Input: part model. Units: mm. Frame: model coordinates. A direction names the side the tool comes from. Coordinates: 2 decimals unless noted, no trailing zeros. Order: outer loops, then holes, each group sorted by start corner. A loop starts at its lowest first (then second) coordinate and runs counter-clockwise, first axis right, second up. Notation, with made-up numbers: M 88.5,61.5 L 119.5,61.5 A19 cw 119.5,91.5 Z; hole C -31.75,89.25 d6. An arc over 180 degrees is marked long. Answer in a Markdown table with one row per item.
from build123d import *

# Parameters (mm, degrees)
PAD_DEPTH       = 12
SKETCH001_R     = 3
HOLE_DEPTH      = 13.001
PAD001_DEPTH    = 7
SKETCH003_W     = 29
SKETCH003_H     = 3
POCKET_DEPTH    = 6
SKETCH004_W     = 29
SKETCH004_H     = 3
POCKET001_DEPTH = 6
SKETCH005_W     = 22
SKETCH005_H     = 10.958168
POCKET002_DEPTH = 6
SKETCH006_W     = 1.8213907522
SKETCH006_H     = 3
POCKET003_DEPTH = 5
SKETCH007_W     = 1.8213907522
SKETCH007_H     = 3
POCKET004_DEPTH = 5


with BuildPart() as part:
    # Sketch → Pad (new body)
    with BuildSketch(Plane.XY):
        Polygon((-20, -10.0810480488), (7.2, -10.0810480488), (7.2, 2.9189519512), (0, 2.9189519512), (0, -7.0810480488), (-20, -7.0810480488), align=None)
    extrude(amount=PAD_DEPTH)

    # Sketch001 (on Face1 of Pad) → Hole (cut, through all)
    with BuildSketch(Plane.XZ.offset(10.0810480488)):
        with Locations((-10, 6)):
            Circle(SKETCH001_R)
    extrude(amount=-HOLE_DEPTH, mode=Mode.SUBTRACT)

    # Sketch002 → Pad001 (join)
    with BuildSketch(Plane.XZ.offset(-2.9)):
        Polygon((37.7, 7.7), (37.7, 0), (0, 0), (0, 11.991246), (0, 65.4), (37.7, 65.4), (37.7, 57.7), (7.7, 57.7), (7.7, 7.7), align=None)
    extrude(amount=PAD001_DEPTH)

    # Sketch003 (on Face15 of Pad001) → Pocket (cut)
    with BuildSketch(Plane(origin=(0, 6, 2.7), x_dir=(1, 0, 0), z_dir=(0, 0, -1))):
        with Locations((21.3996930994, 6.1)):
            Rectangle(SKETCH003_W, SKETCH003_H)
    extrude(amount=-POCKET_DEPTH, mode=Mode.SUBTRACT)

    # Sketch004 (on Face17 of Pocket) → Pocket001 (cut)
    with BuildSketch(Plane(origin=(54, -65, 62.9), x_dir=(1, 0, 0), z_dir=(0, 0, 1))):
        with Locations((-32.6213907522, 64.9)):
            Rectangle(SKETCH004_W, SKETCH004_H)
    extrude(amount=-POCKET001_DEPTH, mode=Mode.SUBTRACT)

    # Sketch005 → Pocket002 (cut)
    with BuildSketch(Plane.XZ.offset(1)):
        with Locations((22.7, 62.096554)):
            Rectangle(SKETCH005_W, SKETCH005_H)
    extrude(amount=-POCKET002_DEPTH, mode=Mode.SUBTRACT)

    # Sketch006 → Pocket003 (cut)
    with BuildSketch(Plane.XY.offset(5.4)):
        with Locations((36.7893046239, -0.1)):
            Rectangle(SKETCH006_W, SKETCH006_H)
    extrude(amount=POCKET003_DEPTH, mode=Mode.SUBTRACT)

    # Sketch007 → Pocket004 (cut)
    with BuildSketch(Plane.XY.offset(61.4)):
        with Locations((36.7893046239, -0.1)):
            Rectangle(SKETCH007_W, SKETCH007_H)
    extrude(amount=-POCKET004_DEPTH, mode=Mode.SUBTRACT)


solid = part.part
1) Material intervals for probe 1 along Z at (x, y) = (14.5, -3.5); probe 2 along Z at (x, y) = (-10, -8.7); probe 3 along Y at (x, z) = (4, 16.5), sorted ascending.
Resolved:
| item | result |
|---|---|
| probe 1 | z = 0 to 7.7, 57.7 to 65.4 |
| probe 2 | z = 0 to 3, 9 to 12 |
| probe 3 | y = -4.1 to 2.9 |
2) Cut plane A-A, the plane x = 12.5. Output: boundary loops of the cut face in (y, z).
Resolved:
| item | result |
|---|---|
| outline | M -4.1,0 L 2.9,0 L 2.9,7.7 L 1.4,7.7 L 1.4,2.7 L -1.6,2.7 L -1.6,7.7 L -4.1,7.7 Z; M -4.1,57.7 L -1.6,57.7 L -1.6,62.9 L -1,62.9 L -1,65.4 L -4.1,65.4 Z |
3) Cut plane C-C, the plane y = -2.5. Output: boundary loops of the cut face in (x, z).
Resolved:
| item | result |
|---|---|
| outline | M 0,0 L 37.7,0 L 37.7,7.7 L 7.7,7.7 L 7.7,57.7 L 37.7,57.7 L 37.7,65.4 L 0,65.4 Z |
4) Cut plane B-B, the plane z = 4. State how many separate pieces and enclosed holes the cut face has, and give its area (3 significant figures).
Resolved:
| item | result |
|---|---|
| separate pieces | 2 |
| enclosed holes | 1 |
| area | 267 mm2 |
5) Contact query for flat-ended pins moving along their axis: pin 1 (1.2 mm diameter, centred on y = 1, z = 60.5, fed in from -X); pin 2 (3.5 mm diameter, centred on x = 19.5, y = 0.5, fed in from +Z); pin 3 (4 mm diameter, centred on x = -1.5, z = 38.5, fed in from -Y); pin 4 (3.5 mm diameter, centred on y = 0, z = 43, fed in from +X). Output: stop coordinate, or through.
Resolved:
| item | result |
|---|---|
| pin 1 | stops at x = 0 |
| pin 2 | stops at z = 65.4 |
| pin 3 | stops at y = -4.1 |
| pin 4 | stops at x = 7.7 |
6) Mould query, pull axis Y, two halves, no side actions, for faces 6 (the face through (0, -1, 33)), 7 (the face through (22, 1.4, 5)), 8 (the face through (-12, -7.081, 3)), 9 (the face through (36, 1.4, 60)). Classes: +Y half, -Y half, draft (parallel to the pull), parting line (faces both ways), or undercut.
Resolved:
| item | result |
|---|---|
| face 6 | draft |
| face 7 | undercut |
| face 8 | +Y half |
| face 9 | undercut |
7) Reachability of faces 1 (the face through (-4, -8, 12)), 2 (the face through (22, -3, 7.7)), 3 (the face through (37.7, -1, 62)), 4 (the face through (35.879, 0, 62)), 5 (the face through (11.7, 2, 62)) from +Z, -Z, +X, -X, +Y, -Y: full face, straight path, thin tool, end or side. Return the list, or none.
Resolved:
| item | result |
|---|---|
| face 1 | +Z, +X, -X, -Y |
| face 2 | +X, +Y, -Y |
| face 3 | +Z, -Z, +X, +Y, -Y |
| face 4 | none |
| face 5 | +Z, +Y |
8) Cut plane D-D, the plane x = -10. Output: boundary loops of the cut face in (y, z).
Resolved:
| item | result |
|---|---|
| outline | M -10.08,0 L -7.08,0 L -7.08,3 L -10.08,3 Z; M -10.08,9 L -7.08,9 L -7.08,12 L -10.08,12 Z |
